Input: part model. Units: mm. Frame: model coordinates. A direction names the side the tool comes from. Give positions to 0.01 mm unless a question says otherwise; leave off trailing zeros. Loops run counter-clockwise (first coordinate to the right, second up) from the corner with the lowest first, then second, coordinate; pieces in that order, holes last.
from build123d import *

# Parameters (mm, degrees)
SKETCH1_R               = 15
SKETCH1_R_2             = 4.6
BOSS_EXTRUDE1_DEPTH     = 14
SKETCH2_W               = 12.4
SKETCH2_H               = 1.2
CUT_EXTRUDE1_DEPTH      = 26.416530054
CUT_EXTRUDE2_DEPTH      = 26.416530054
CUT_EXTRUDE2_DEPTH_BACK = 26.416530054
SKETCH3_R               = 2
CUT_EXTRUDE3_REACH      = 30.306
CUT_EXTRUDE3_END_RADIUS = 15
SKETCH4_R               = 3.6
CUT_EXTRUDE4_REACH      = 30.306
CUT_EXTRUDE4_END_RADIUS = 15


with BuildPart() as part:
    # Sketch1 → Boss-Extrude1 (new body)
    with BuildSketch(Plane.XY):
        Circle(SKETCH1_R)
        Circle(SKETCH1_R_2, mode=Mode.SUBTRACT)
    extrude(amount=BOSS_EXTRUDE1_DEPTH)

    # Sketch2 → Cut-Extrude1 (cut, through all)
    with BuildSketch(Plane.XY.offset(14)):
        with Locations((9.8, 0)):
            Rectangle(SKETCH2_W, SKETCH2_H)
    extrude(amount=-CUT_EXTRUDE1_DEPTH, mode=Mode.SUBTRACT)

    # Sketch3 → Cut-Extrude2 (cut, two sides: drawn at the far end of the back side and taken through both)
    with BuildSketch(Plane(origin=(0, 0, 0), x_dir=(1, 0, 0), z_dir=(0, 1, 0)).offset(-CUT_EXTRUDE2_DEPTH_BACK)):
        with Locations(Location((9.774348448, -7, 0), (0, 0, 270))):
            Circle(SKETCH3_R)
    extrude(amount=CUT_EXTRUDE2_DEPTH + CUT_EXTRUDE2_DEPTH_BACK, mode=Mode.SUBTRACT)

    # Cut-Extrude3: up to this cylinder (the profile starts inside it)
    cut_extrude3_end = Plane(origin=(0, 0, 7), z_dir=(0, 0, -1)) * Cylinder(CUT_EXTRUDE3_END_RADIUS, 91.612, mode=Mode.PRIVATE)
    # Sketch4 → Cut-Extrude3 (cut, up to the surface)
    with BuildSketch(Plane(origin=(0, 4.5, 0), x_dir=(1, 0, 0), z_dir=(0, 1, 0)), mode=Mode.PRIVATE) as cut_extrude3_sk1:
        with Locations(Location((9.774348448, -7, 0), (0, 0, 90))):
            Circle(SKETCH4_R)
    cut_extrude3_tool1 = extrude(cut_extrude3_sk1.sketch, amount=CUT_EXTRUDE3_REACH, mode=Mode.PRIVATE) & cut_extrude3_end
    add(cut_extrude3_tool1.solids().sort_by_distance((9.774348, 4.5, 7))[0], mode=Mode.SUBTRACT)

    # Cut-Extrude4: up to this cylinder (the profile starts inside it)
    cut_extrude4_end = Plane(origin=(0, 0, 7), z_dir=(0, 0, -1)) * Cylinder(CUT_EXTRUDE4_END_RADIUS, 91.612, mode=Mode.PRIVATE)
    # Sketch5 → Cut-Extrude4 (cut, up to the surface)
    with BuildSketch(Plane(origin=(0, -4.5, 0), x_dir=(1, 0, 0), z_dir=(0, 1, 0)), mode=Mode.PRIVATE) as cut_extrude4_sk1:
        Polygon((6.229720914, -9.058870802), (9.785069099, -11.099172892), (13.329696633, -9.04030209), (13.318975982, -4.941129198), (9.763627798, -2.900827108), (6.219000264, -4.95969791), align=None)
    cut_extrude4_tool1 = extrude(cut_extrude4_sk1.sketch, amount=-CUT_EXTRUDE4_REACH, mode=Mode.PRIVATE) & cut_extrude4_end
    add(cut_extrude4_tool1.solids().sort_by_distance((9.774348, -4.5, 7))[0], mode=Mode.SUBTRACT)


solid = part.part
(1) Cut plane B-B (z = 7). Return the cut outline in (x, y).
Values follow:
outline: (4.56, -0.6) arc R4.6 cw (long way) to (4.56, 0.6) - (7.77, 0.6) - (7.77, 4.5) - (6.17, 4.5) - (6.17, 13.67) arc R15 ccw (long way) to (6.22, -13.65) - (6.22, -4.5) - (7.77, -4.5) - (7.77, -0.6) - close; (11.77, -4.5) - (13.32, -4.5) - (13.32, -6.89) arc R15 ccw to (14.99, -0.6) - (11.77, -0.6) - close; (11.77, 0.6) - (14.99, 0.6) arc R15 ccw to (13.37, 6.79) - (13.37, 4.5) - (11.77, 4.5) - close
(2) Cut plane D-D (y = -6). Return the cut outline in (x, z), and give its area (3 significant figures).
Values follow:
outline: (-13.75, 0) - (13.75, 0) - (13.75, 14) - (-13.75, 14) - close; hole (6.22, 4.96) - (9.76, 2.9) - (13.32, 4.94) - (13.33, 9.04) - (9.79, 11.1) - (6.23, 9.06) - close
area: 341 mm2
(3) Reachability of faces 4 (the cylindrical face through (6.205, 8.002, 7.469)), 5 (the flat face through (8.016, -9.011, 3.916)), 6 (the cylindrical face through (7.82, -2.58, 6.57)), 7 (the flat face through (7, 0.6, 7)), 8 (the flat face through (-4, -3, 0)) from +Z, -Z, +X, -X, +Y, -Y: full face, straight path, thin tool, end or side. Return the list, or none.
Values follow:
face 4: +Y
face 5: -Y
face 6: +Y, -Y
face 7: +Z, -Z, +X
face 8: -Z, +X, -X, +Y, -Y
(4) Cut plane C-C (x = 0). Return the cut outline in (y, z), and give its area (3 significant figures).
Values follow:
outline: (-15, 0) - (-4.6, 0) - (-4.6, 14) - (-15, 14) - close; (4.6, 0) - (15, 0) - (15, 14) - (4.6, 14) - close
area: 291 mm2
(5) Pin query (flat end, axial travel): pin 1 Ø6 at (x, y) = (2, -4.5) entering from -Z; pin 2 Ø4 at (y, z) = (-12, 5) entering from -X; pin 3 Ø6.5 at (x, z) = (9.77, 7) entering from -Y; pin 4 Ø5 at (x, z) = (6.5, 5) entering from +Y. Return the tip coordinate at first contact, or that it passes through.
Values follow:
pin 1: stops at z = 0
pin 2: stops at x = -11.18
pin 3: stops at y = -4.5
pin 4: stops at y = 14.46
(6) Ray query, probe 1 along Y at (x, z) = (11.5, 9); probe 2 along Y at (x, z) = (0, 5.5); probe 3 along X at (y, z) = (-2, 6.25). Return the intervals inside material, ascending.
Values follow:
probe 1: y = -4.5 to -0.6, 0.6 to 4.5
probe 2: y = -15 to -4.6, 4.6 to 15
probe 3: x = -14.87 to -4.14, 4.14 to 7.92, 11.63 to 14.87
(7) Mould query, pull axis Y, two halves, no side actions, for faces 1 (the flat face through (11.14, -7.12, 10.31)), 2 (the flat face through (11, -4.5, 5)), 3 (the flat face through (7, -0.6, 7)). Classes: +Y half, -Y half, draft (parallel to the pull), parting line (faces both ways), or undercut.
Values follow:
face 1: draft
face 2: -Y half
face 3: undercut
(8) Cut plane A-A (y = 1). Return the cut outline in (x, z).
Values follow:
outline: (-14.97, 0) - (-4.49, 0) - (-4.49, 14) - (-14.97, 14) - close; (4.49, 0) - (14.97, 0) - (14.97, 14) - (4.49, 14) - close; hole circle Ø4 at (9.77, 7)
